Design review of the part shown in the three views and the two pictorial views. Dimensions are in mm from the part's minimum x, y and z. Round coordinates to 2 decimals unless told otherwise and drop trailing zeros. Write each loop counter-clockwise with the first axis right and the second up, starting at its lowest first coordinate (ties: lowest second). Pieces come first, ordered by that corner, then holes. Notation, with made-up numbers: (-14.5, 53) -> (34.5, 53) arc R10 ccw to (34.5, 65) -> close; hole circle Ø2 at (-33, 40.25). An arc over 180 degrees is marked (long way). Answer as a JSON object with one key per item and string values. Group by question number.
1) We need section A-A, the plane x = 90.5. Write out the cut boundary in (y, z), then the cut area to 3 significant figures.
2) To check wall thickness, follow probe 1 along Y at (x, z) = (903, 44). State the ranges of the line that lie inside material, in increasing order. Write a range as [from, to].
3) Insertion check: pin 1 Ø12 at (x, y) = (503, 50) entering from -Z; pin 2 Ø10 at (x, z) = (519, 60) entering from +Y; pin 3 Ø24 at (x, y) = (339, 55) entering from +Z. Each pin has a flat end and moves straight along its axis. Give the tip position at first contact, or say it passes through.
4) We need section B-B, the plane y = 36.5. Write out the cut boundary in (x, z).
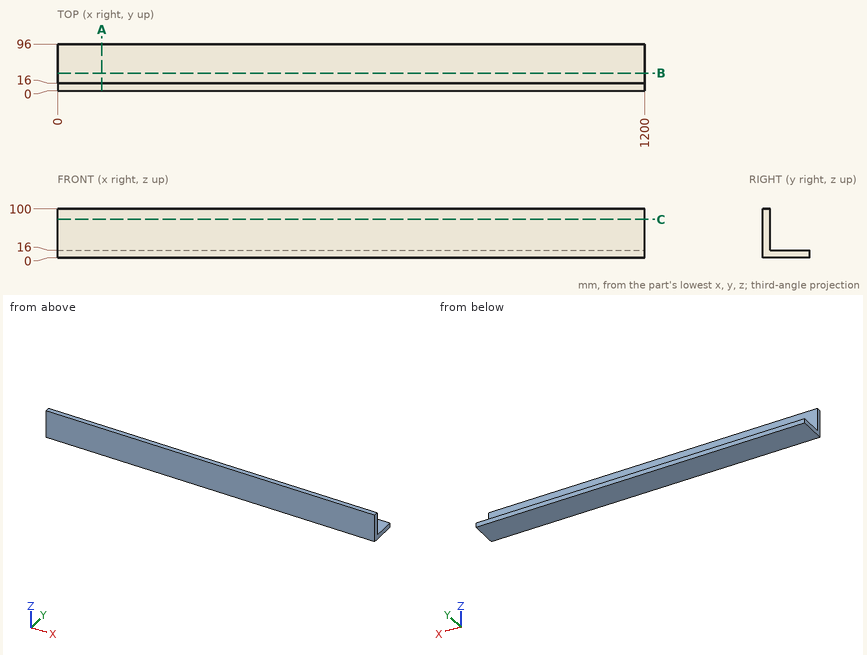
Here are the results:
{
 "1": {"outline": "(0, 0) -> (96, 0) -> (96, 16) -> (16, 16) -> (16, 100) -> (0, 100) -> close", "area": "2,880 mm^2"},
 "2": {"probe 1": "y = [0, 16]"},
 "3": {"pin 1": "stops at z = 0", "pin 2": "stops at y = 16", "pin 3": "stops at z = 16"},
 "4": {"outline": "(0, 0) -> (1200, 0) -> (1200, 16) -> (0, 16) -> close"}
}
